CAD build for the part. Positions are in the model's coordinates, mm. A direction names the side the tool comes from. Coordinates: 2 decimals unless noted, no trailing zeros. Order: outer loops, then holes, each group sorted by start corner. A loop starts at its lowest first (then second) coordinate and runs counter-clockwise, first axis right, second up. Notation, with made-up numbers: (-37, 84) - (-23, 84) arc R24 ccw to (-23, 105) - close; hole circle Ø2 at (-36, -27). An arc over 180 degrees is marked (long way). Return JSON: item names as keys, results as strings.
from build123d import *

# Parameters (mm, degrees)
F1_DEPTH  = 6
F0_W      = 8
F0_H      = 52
F2_DEPTH  = 3
F0_W_2    = 98
F0_H_2    = 92.5
F3_DEPTH  = 32
F5_W      = 28
F5_H      = 5
F6_DEPTH  = 20
F0_W_3    = 95
F0_H_3    = 23.5
F0_R      = 2
F0_R_2    = 6
F0_R_3    = 4
F7_DEPTH  = 2.25
F9_W      = 105
F9_H      = 99.5
F9_W_2    = 95
F9_H_2    = 89.5
F10_DEPTH = 3
F11_SIZE  = 3.49999
F12_R     = 1


# Not quite as in the source:
# - a fillet or chamfer is up to 0.001 mm smaller than in the source, because OpenCascade refuses the exact size
# - a feature names something its author has since deleted; it is built from what else it names


with BuildPart() as f1:
    # F0 (on Top) → F1 (new body)
    with BuildSketch(Plane.XY):
        Polygon((0, 52), (0, 0), (-79, 0), (-87, 0), (-87, -3), (8, -3), (8, 63), (-87, 63), (-87, 52), (-79, 52), align=None)
    extrude(amount=-F1_DEPTH)

    # F0 (on Top) → F2 (join)
    with BuildSketch(Plane.XY):
        with Locations((-83, 26)):
            Rectangle(F0_W, F0_H)
    extrude(amount=-F2_DEPTH)

    # F0 (on Top) → F3 (join)
    with BuildSketch(Plane.XY):
        with Locations((-39.5, 18.25)):
            Rectangle(F0_W_2, F0_H_2)
        Polygon((-87, -3), (-87, 0), (-87, 52), (-87, 63), (8, 63), (8, -3), (8, -26.5), (-87, -26.5), align=None, mode=Mode.SUBTRACT)
    extrude(amount=-F3_DEPTH)

    # F5 (on offset) → F6 (cut)
    with BuildSketch(Plane.YZ.offset(-88.5)):
        with Locations((26, -15.5)):
            Rectangle(F5_W, F5_H)
    extrude(amount=F6_DEPTH, mode=Mode.SUBTRACT)

    # F0 (on Top) → F7 (join)
    with BuildSketch(Plane.XY):
        with Locations((-39.5, -14.75)):
            Rectangle(F0_W_3, F0_H_3)
        with Locations((-37, -18)):
            Circle(F0_R, mode=Mode.SUBTRACT)
        with Locations((-21, -18)):
            Circle(F0_R_2, mode=Mode.SUBTRACT)
        with Locations((-3, -18)):
            Circle(F0_R_3, mode=Mode.SUBTRACT)
    extrude(amount=-F7_DEPTH)

    # F9 (on offset) → F10 (join)
    with BuildSketch(Plane.XY.offset(-32)):
        with Locations((-39.5, 18.25)):
            Rectangle(F9_W, F9_H)
        with Locations((-39.5, 18.25)):
            Rectangle(F9_W_2, F9_H_2, mode=Mode.SUBTRACT)
    extrude(amount=F10_DEPTH)

    # F11 (size 3.5 in the source; OpenCascade refuses exactly that, so slightly less here)
    f11_edges = [f1.edges().sort_by_distance(p)[0] for p in [
        (-88.5, 18.25, -29),
        (-39.5, -28, -29),
        (9.5, 18.25, -29),
        (-39.5, 64.5, -29),
    ]]
    chamfer(f11_edges, length=F11_SIZE)

    # F12
    f12_edges = [f1.edges().sort_by_distance(p)[0] for p in [
        (-88.5, -28, -12.750005),
        (-39.5, -28, 0),
        (-88.5, 18.25, 0),
        (-39.5, 64.5, 0),
        (9.5, 18.25, 0),
        (0, 26, 0),
        (-39.5, 0, 0),
        (-79, 26, 0),
        (-39.5, 52, 0),
        (9.5, -28, -12.750005),
        (9.5, 64.5, -12.750005),
        (-88.5, 64.5, -12.750005),
    ]]
    fillet(f12_edges, radius=F12_R)


solid = f1.part
Item 1: Wall check: L1, parallel to Y at x = -51.5, z = -3.5; L2, parallel to Y at x = -37, z = -1.3; L3, parallel to Y at x = -21.5, z = -20. Give the ranges that are in metal, low to high. Write a range as [from, to].
Findings below:
{"L1": "y = [-28, -26.5], [-3, 0], [52, 64.5]", "L2": "y = [-28, -20], [-16, 0], [52, 64.5]", "L3": "y = [-28, -26.5], [63, 64.5]"}
Item 2: Band-saw the part on A-A, the plane x = -3. Count the separate pieces of the cut face and the enclosed holes in it, then the cut area to 3 significant figures.
Findings below:
{"separate pieces": "3", "enclosed holes": "0", "area": "247 mm²"}
Item 3: Mould opens along Y. For faces 1 (the flat face through (0, 26, -3)), 2 (the flat face through (-40.2, -1.2, 0)), 3 (the flat face through (-40, -31.5, -31)) say: released by +Y, released by -Y, zero draft, split by the parting line, or undercut.
Findings below:
{"face 1": "undercut", "face 2": "zero draft", "face 3": "released by -Y"}
Item 4: Band-saw the part on C-C, the plane z = -10.5. List the corners of the cut face in (x, y), then the cut area to 3 significant figures.
Findings below:
{"outline": "(-88.5, -27) arc R1 ccw to (-87.5, -28) - (8.5, -28) arc R1 ccw to (9.5, -27) - (9.5, 63.5) arc R1 ccw to (8.5, 64.5) - (-87.5, 64.5) arc R1 ccw to (-88.5, 63.5) - close; hole (-87, -26.5) - (8, -26.5) - (8, 63) - (-87, 63) - close", "area": "562 mm²"}
Item 5: Drop flat-ended pins along their axis: P1, Ø6, axis at x = -72.5, z = -10.5, coming from the -Y side; P2, Ø1, axis at x = -39.5, z = -19.5, coming from the +Y side; P3, Ø1.5, axis at y = 50.5, z = -15.5, coming from the +X side; P4, Ø3, axis at x = -37, y = -18, coming from the +Z side. Give the stop position or say it passes through.
Findings below:
{"P1": "stops at y = -28", "P2": "stops at y = 64.5", "P3": "stops at x = 9.5", "P4": "passes through"}
Item 6: Which spindle directions (+Z, -Z, +X, -X, +Y, -Y) get a long thin tool onto all of the face, cutting with end or side? Do faces 4 (the flat face through (-40, -3, -4)), 5 (the flat face through (13, 18, -31)). Say none if no direction does.
Findings below:
{"face 4": "-Z", "face 5": "+Z, -Z, +X, +Y, -Y"}
